Answer from the drawing. Dimensions are ordinates in mm from the lowest x, y and z of the part. A direction names the side the tool comes from. Coordinates: 2 decimals unless noted, no trailing zeros. Write each loop counter-clockwise with the first axis right and the second up, starting at its lowest first coordinate (ties: lowest second). Pieces come first, ordered by that corner, then holes. Notation, with made-up numbers: (-15, 18) - (19, 18) arc R15 ccw to (19, 25) - close; hole circle Ø11 at (39.25, -26). An arc over 180 degrees is marked (long way). Use a Markdown table: item, result.
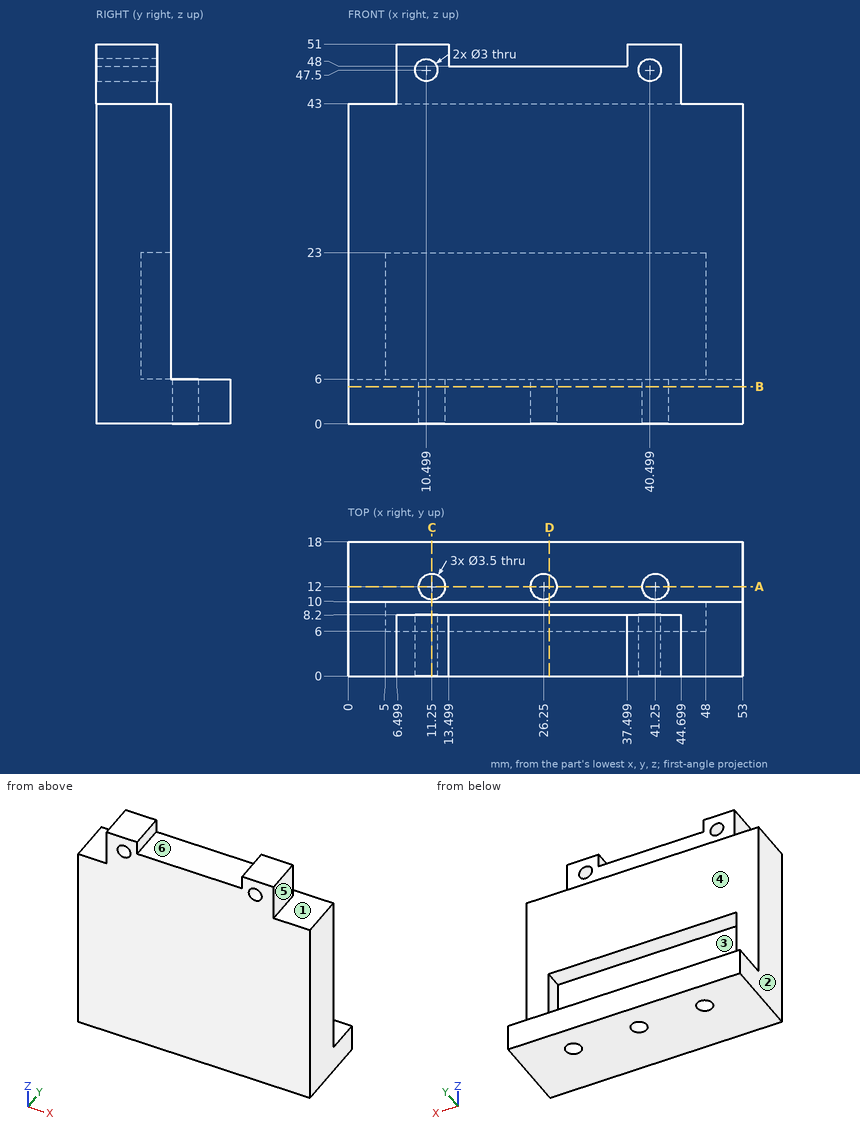
(1) A cutting plane is placed at B-B, the plane z = 5. Write down the section's boundary in (x, y).
Report:
| item | result |
|---|---|
| outline | (0, 0) - (53, 0) - (53, 18) - (0, 18) - close; hole circle Ø3.5 at (11.25, 12); hole circle Ø3.5 at (26.25, 12); hole circle Ø3.5 at (41.25, 12) |
(2) The mould has two halves that part along X. Classify the marked faces 1, 2 and 3: pulls with the +X half, pulls with the -X half, needs draft (parallel to the pull), parting line crosses it, or undercut.
Report:
| item | result |
|---|---|
| face 1 | needs draft |
| face 2 | pulls with the -X half |
| face 3 | undercut |
(3) Each of these flat-tipped pins is pushed along its axis until it touches: P1, Ø4, axis at x = 25, z = 47.5, coming from the +Y side; P2, Ø4, axis at x = 37.5, z = 22.5, coming from the +Y side; P3, Ø6.5, axis at x = 30, y = 2.5, coming from the +Z side. Where does it stop, or does it pass through?
Report:
| item | result |
|---|---|
| P1 | stops at y = 8.2 |
| P2 | stops at y = 10 |
| P3 | stops at z = 48 |
(4) A cutting plane is placed at C-C, the plane x = 11.25. Write down the section's boundary in (y, z).
Report:
| item | result |
|---|---|
| outline | (0, 0) - (10.25, 0) - (10.25, 6) - (6, 6) - (6, 23) - (10, 23) - (10, 43) - (8.2, 43) - (8.2, 46.2) - (0, 46.2) - close; (0, 48.8) - (8.2, 48.8) - (8.2, 51) - (0, 51) - close; (13.75, 0) - (18, 0) - (18, 6) - (13.75, 6) - close |
(5) A cutting plane is placed at A-A, the plane y = 12. Write down the section's boundary in (x, z), and give its area (3 significant figures).
Report:
| item | result |
|---|---|
| outline | (0, 0) - (9.5, 0) - (9.5, 6) - (0, 6) - close; (13, 0) - (24.5, 0) - (24.5, 6) - (13, 6) - close; (28, 0) - (39.5, 0) - (39.5, 6) - (28, 6) - close; (43, 0) - (53, 0) - (53, 6) - (43, 6) - close |
| area | 255 mm² |
(6) For the marked faces 4, 5 and 6, determine the directions among +Z, -Z, +X, -X, +Y, -Y from which every point of the face is accessible in a straight line to the end or side of a thin tool.
Report:
| item | result |
|---|---|
| face 4 | +Z, +X, -X, +Y |
| face 5 | +Z, +X, +Y, -Y |
| face 6 | +Z, +Y, -Y |
(7) A cutting plane is placed at D-D, the plane x = 27. Write down the section's boundary in (y, z), and give its area (3 significant figures).
Report:
| item | result |
|---|---|
| outline | (0, 0) - (10.42, 0) - (10.42, 6) - (6, 6) - (6, 23) - (10, 23) - (10, 43) - (8.2, 43) - (8.2, 48) - (0, 48) - close; (13.58, 0) - (18, 0) - (18, 6) - (13.58, 6) - close |
| area | 432 mm² |
(8) Straight lines are drawn through the part: L1, parallel to X at y = 6, z = 47.5; L2, parallel to Z at x = 34.5, y = 8.75; L3, parallel to Z at x = 26, y = 6.25. For each, find the intervals that lie inside material, in ascending order.
Report:
| item | result |
|---|---|
| L1 | x = 6.5 to 9, 12 to 39, 42 to 44.7 |
| L2 | z = 0 to 6, 23 to 43 |
| L3 | z = 0 to 6, 23 to 48 |
